For this review, take the finished solid that the model builds, in its own axes (mm). A direction names the side the tool comes from. Coordinates: 2 decimals unless noted, no trailing zeros. Loops run counter-clockwise (first coordinate to the right, second up) from the corner with the lowest first, then second, coordinate; pieces in that order, holes last. Notation, with made-up numbers: (-19.5, 82.25) - (12.5, 82.25) arc R14 cw to (12.5, 94.25) - close; hole circle Ø7 at (38.25, 85). An arc over 180 degrees is marked (long way). One line per item, written item: value. Start each with the question number.
1. Insertion check: pin 1 (1 mm diameter, centred on y = 32, z = 0, fed in from -X); pin 2 (0.6 mm diameter, centred on x = -51, z = 0, fed in from -Y); pin 3 (0.6 mm diameter, centred on x = -42, z = 0.5, fed in from -Y). Each pin has a flat end and moves straight along its axis. Give the tip position at first contact, or say it passes through.
2. Take a section at C-C, the plane x = 16. State the section outline as (y, z) points.
3. Take a section at B-B, the plane y = -22. State the section outline as (x, z) points, and give its area (3 significant figures).
4. To check wall thickness, follow line 1 (X direction, y = 19, z = -0.9); line 2 (X direction, y = 33.5, z = 0.3); line 3 (Y direction, x = -58, z = -0.5). State the ranges of each line that lie inside material, in increasing order. Write a range as from..to.
5. The part is to be moulded in two halves that separate along X. For faces 6 (the face through (-60, -29.6, 0)), 7 (the face through (-68.011, 18, 0)), 8 (the face through (-70.411, -18, 0)), say which applies: released by +X, released by -X, zero draft, split by the parting line, or undercut.
6. Take a section at A-A, the plane x = -63. State the section outline as (y, z) points, and give its area (3 significant figures).
7. For faces 1 (the face through (-69.211, 0, 0)), 2 (the face through (-52.611, 22, 0)), 3 (the face through (-45.711, 20, 0)), 4 (the face through (-27, 17, -1)), 5 (the face through (-50.211, -27, 0)), list the 3-axis set-ups (+Z, -Z, +X, -X, +Y, -Y) from which the entire face can be reached by the end or side of a thin tool; tool diameter is ignored.
```python
from build123d import *

# Parameters (mm, degrees)
F1_DEPTH = 1


with BuildPart() as f1:
    # F0 (on Top) → F1 (new body, symmetric)
    with BuildSketch(Plane.XY):
        with BuildLine():
            Line((-70.4106393839, -7.0998651044), (-70.4106393839, -29.5998683792))
            Line((-70.4106393839, -29.5998683792), (-50.2106361091, -29.5998683792))
            Line((-50.2106361091, -29.5998683792), (-50.2106361091, -23.339858427))
            Line((-50.2106361091, -23.339858427), (-9.3698940826, -34.4484426613))
            ThreePointArc((-9.3698940826, -34.4484426613), (20.713103481, -29.0767512129), (35.6192379066, -2.4000016374))
            Line((35.6192379066, -2.4000016374), (41.13003923, -2.4000016374))
            ThreePointArc((41.13003923, -2.4000016374), (39.8466372276, 10.4730910707), (34.6344497709, 22.3135614366))
            Line((34.6344497709, 22.3135614366), (27.8674558028, 22.3135614366))
            ThreePointArc((27.8674558028, 22.3135614366), (22.9275534697, 27.3645282949), (17.0897025746, 31.3437742274))
            Line((17.0897025746, 31.3437742274), (17.0897025746, 37.1873599962))
            Line((17.0897025746, 37.1873599962), (-23.7103007001, 37.1873599962))
            Line((-23.7103007001, 37.1873599962), (-23.7103007001, 28.1873608961))
            Line((-23.7103007001, 28.1873608961), (-25.7103007001, 28.1873608961))
            Line((-25.7103007001, 28.1873608961), (-25.7103007001, 18.6000016374))
            Line((-25.7103007001, 18.6000016374), (-45.7106326896, 18.6000016374))
            Line((-45.7106326896, 18.6000016374), (-45.7106326896, 20.6000016374))
            Line((-45.7106326896, 20.6000016374), (-50.2106326896, 20.6000016374))
            Line((-50.2106326896, 20.6000016374), (-50.2106326896, 28.6000016374))
            Line((-50.2106326896, 28.6000016374), (-70.4106393839, 28.6000016374))
            Line((-70.4106393839, 28.6000016374), (-70.4106393839, 7.0999983626))
            Line((-70.4106393839, 7.0999983626), (-69.2106393839, 7.0999983626))
            Line((-69.2106393839, 7.0999983626), (-69.2106393839, 1.4001348956))
            Line((-69.2106393839, 1.4001348956), (-69.2106393839, -7.0998651044))
            Line((-69.2106393839, -7.0998651044), (-70.4106393839, -7.0998651044))
        make_face()
        with BuildLine():
            ThreePointArc((33.3, 0), (20.2218755926, -26.4568657916), (-8.7399848359, -32.132579496))
            Line((-8.7399848359, -32.132579496), (-52.6106377465, -20.1998667418))
            Line((-52.6106377465, -20.1998667418), (-52.6106377465, -27.1998667418))
            Line((-52.6106377465, -27.1998667418), (-68.0106377465, -27.1998667418))
            Line((-68.0106377465, -27.1998667418), (-68.0106377465, -9.4998667418))
            Line((-68.0106377465, -9.4998667418), (-66.8106377465, -9.4998667418))
            Line((-66.8106377465, -9.4998667418), (-66.8106377465, -0.9998667418))
            Line((-66.8106377465, -0.9998667418), (-65.8106377465, -0.9998667418))
            Line((-65.8106377465, -0.9998667418), (-65.8106377465, 0))
            Line((-65.8106377465, 0), (-65.8106377465, 1))
            Line((-65.8106377465, 1), (-66.8106377465, 1))
            Line((-66.8106377465, 1), (-66.8106377465, 9.5))
            Line((-66.8106377465, 9.5), (-68.0106377465, 9.5))
            Line((-68.0106377465, 9.5), (-68.0106377465, 26.2))
            Line((-68.0106377465, 26.2), (-52.6106343269, 26.2))
            Line((-52.6106343269, 26.2), (-52.6106343269, 18.2))
            Line((-52.6106343269, 18.2), (-48.1106343269, 18.2))
            Line((-48.1106343269, 18.2), (-48.1106343269, 16.2))
            Line((-48.1106343269, 16.2), (-23.3102990627, 16.2))
            Line((-23.3102990627, 16.2), (-23.3102990627, 25.7873592587))
            Line((-23.3102990627, 25.7873592587), (-21.3102990627, 25.7873592587))
            Line((-21.3102990627, 25.7873592587), (-21.3102990627, 34.7873583588))
            Line((-21.3102990627, 34.7873583588), (14.6897009373, 34.7873583588))
            Line((14.6897009373, 34.7873583588), (14.6897009373, 29.8848236798))
            ThreePointArc((14.6897009373, 29.8848236798), (21.2819230973, 25.6119063969), (26.6897009373, 19.9135597993))
            Line((26.6897009373, 19.9135597993), (33.3000020439, 19.9135597993))
            ThreePointArc((33.3000020439, 19.9135597993), (37.3997331495, 10.3295672876), (38.8, 0))
            Line((38.8, 0), (33.3, 0))
        make_face(mode=Mode.SUBTRACT)
    extrude(amount=F1_DEPTH, both=True)


solid = f1.part
```
Solutions:
1. pin 1: x = -23.71
1. pin 2: y = -29.6
1. pin 3: y = -25.65
2. outline: (-31.91, -1) - (-29.2, -1) - (-29.2, 1) - (-31.91, 1) - close; (29.2, -1) - (37.19, -1) - (37.19, 1) - (29.2, 1) - close
3. outline: (-70.41, -1) - (-68.01, -1) - (-68.01, 1) - (-70.41, 1) - close; (-52.61, -1) - (-45.99, -1) - (-45.99, 1) - (-52.61, 1) - close; (25, -1) - (28.12, -1) - (28.12, 1) - (25, 1) - close
3. area: 24.3 mm2
4. line 1: -70.41..-68.01, -52.61..-45.71, -25.71..-23.31, 33.83..36.56
4. line 2: -23.71..-21.31, 14.69..17.09
4. line 3: -29.6..-27.2, 26.2..28.6
5. face 6: zero draft
5. face 7: undercut
5. face 8: released by -X
6. outline: (-29.6, -1) - (-27.2, -1) - (-27.2, 1) - (-29.6, 1) - close; (26.2, -1) - (28.6, -1) - (28.6, 1) - (26.2, 1) - close
6. area: 9.60 mm2
7. face 1: +Z, -Z, -X
7. face 2: +Z, -Z
7. face 3: +Z, -Z, +Y
7. face 4: -Z, +X, -X, +Y, -Y
7. face 5: +Z, -Z, -Y
